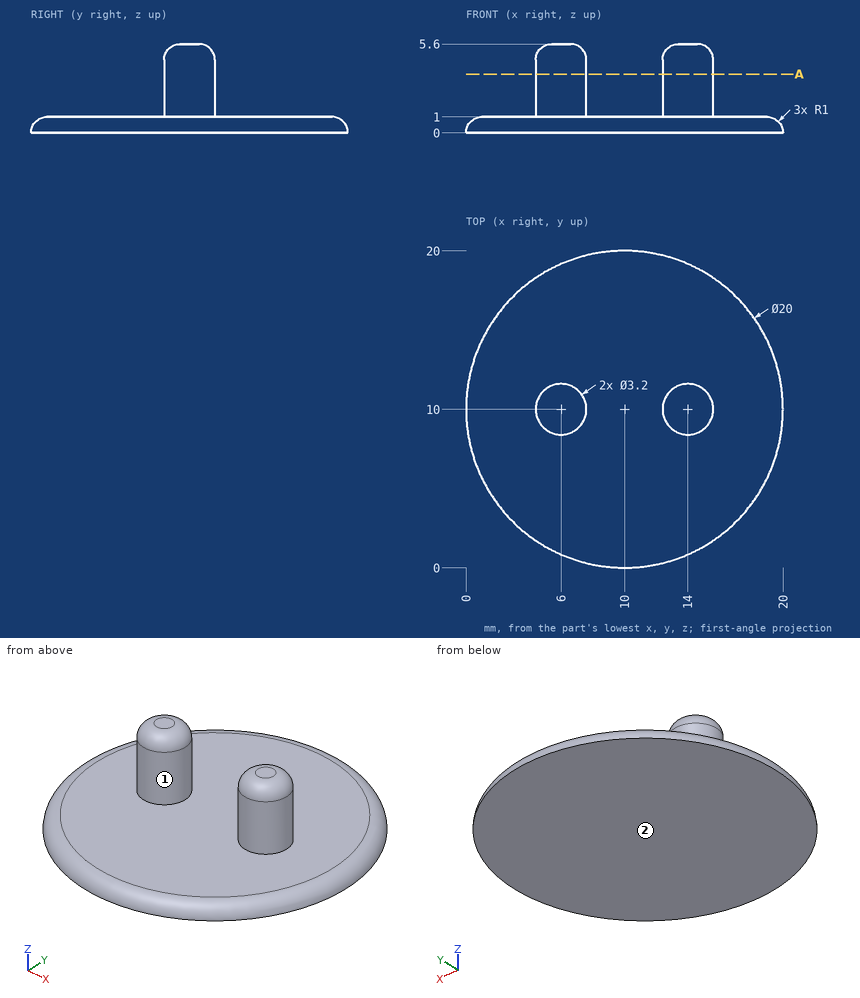
Answer from the drawing. Dimensions are ordinates in mm from the lowest x, y and z of the part. Give positions to 0.01 mm unless a question says otherwise; leave off trailing zeros. Order: outer loops, then holes, each group sorted by start corner. A loop starts at its lowest first (then second) coordinate and runs counter-clockwise, first axis right, second up.
Item 1: Find the intervals of material crossed by probe 1 along Z at (x, y) = (16, 11); probe 2 along Y at (x, z) = (7, 0.9); probe 3 along Z at (x, y) = (14.5, 9), in increasing order.
From the geometry:
probe 1: z = 0 to 1
probe 2: y = 1.05 to 18.95
probe 3: z = 0 to 5.46
Item 2: Given pin 1 Ø1.5 at (y, z) = (6.5, 1) entering from +X; pin 2 Ø1.5 at (x, z) = (12.5, 3.5) entering from +Y, each flat-ended and moving along its own axis, determine where each tip first touches the part or whether it passes through.
From the geometry:
pin 1: stops at x = 19.44
pin 2: stops at y = 11.41
Item 3: For a pull along X with two mould halves and no side action, classify the marked faces 1 and 2 as pulls with the +X half, pulls with the -X half, needs draft (parallel to the pull), parting line crosses it, or undercut.
From the geometry:
face 1: undercut
face 2: needs draft
Item 4: The part is cut by section A-A, the plane z = 3.7. Give the vertices of the cut face in (x, y), and give its area (3 significant figures).
From the geometry:
outline: circle Ø3.2 at (6, 10); circle Ø3.2 at (14, 10)
area: 16.1 mm2
